from build123d import *

# Parameters (mm, degrees)
F0_W         = 298.45
F0_H         = 457.2
F1_DEPTH     = 19.05
F3_W         = 19.05
F3_H         = 457.2
F4_DEPTH     = 6.35
F5_T1_DEPTH  = 327.025
F5_T3_DEPTH  = 419.1
F5_T5_DEPTH  = 47.625
F5_S9_W      = 19.05
F5_S9_H      = 19.05
F5_T10_DEPTH = 19.05
F5_S15_W     = 19.05
F5_S15_H     = 19.05
F5_T16_DEPTH = 19.05
F6_W         = 19.05
F6_H         = 457.2
F7_DEPTH     = 19.05
F8_W         = 76.2
F8_H         = 19.05
F9_DEPTH     = 6.35


# Not quite as in the source:
# - a fillet or chamfer that OpenCascade refuses, or shapes differently, is made with other operations: its cross-section is extruded or revolved along the edge and cut away or added


with BuildPart() as f1:
    # F0 (on Front) → F1 (new body)
    with BuildSketch(Plane.XZ):
        Rectangle(F0_W, F0_H)
    extrude(amount=-F1_DEPTH)

    # F3 (on face) → F4 (cut)
    with BuildSketch(Plane(origin=(0, 19.05, 0), x_dir=(-1, 0, 0), z_dir=(0, 1, 0))):
        with Locations((-114.3, 0)):
            Rectangle(F3_W, F3_H)
    extrude(amount=-F4_DEPTH, mode=Mode.SUBTRACT)

    # F5: fillet of radius 19.05 on 5 edges, made by hand

    # F5_s2 → F5_t1 (cut)
    with BuildSketch(Plane.YZ.offset(-196.85)):
        with BuildLine():
            ThreePointArc((19.05, -228.6), (5.5796158184, -223.0203841816), (0, -209.55))
            Line((0, -209.55), (0, -228.6))
            Line((0, -228.6), (19.05, -228.6))
        make_face()
        with BuildLine():
            ThreePointArc((19.05, 228.6), (5.5796158184, 223.0203841816), (0, 209.55))
            Line((0, 209.55), (0, 228.6))
            Line((0, 228.6), (19.05, 228.6))
        make_face()
    extrude(amount=F5_T1_DEPTH, mode=Mode.SUBTRACT)

    # F5_s4 → F5_t3 (cut)
    with BuildSketch(Plane.XY.offset(-209.55)):
        with BuildLine():
            ThreePointArc((130.175, 0), (143.6453841816, 5.5796158184), (149.225, 19.05))
            Line((149.225, 19.05), (149.225, 0))
            Line((149.225, 0), (130.175, 0))
        make_face()
    extrude(amount=F5_T3_DEPTH, mode=Mode.SUBTRACT)

    # F5_s6 → F5_t5 (cut)
    with BuildSketch(Plane.XZ.offset(-66.675)):
        with BuildLine():
            ThreePointArc((130.175, -228.6), (143.6453841816, -223.0203841816), (149.225, -209.55))
            Line((149.225, -209.55), (149.225, -228.6))
            Line((149.225, -228.6), (130.175, -228.6))
        make_face()
        with BuildLine():
            ThreePointArc((130.175, 228.6), (143.6453841816, 223.0203841816), (149.225, 209.55))
            Line((149.225, 209.55), (149.225, 228.6))
            Line((149.225, 228.6), (130.175, 228.6))
        make_face()
    extrude(amount=F5_T5_DEPTH, mode=Mode.SUBTRACT)


with BuildPart() as f5_tool8:
    # F5_s9 → F5_t10 (new body)
    with BuildSketch(Plane.YZ.offset(130.175)):
        with Locations((9.525, -219.075)):
            Rectangle(F5_S9_W, F5_S9_H)
    extrude(amount=F5_T10_DEPTH)

    # F5_s11 → F5_t12 (revolve, cut)
    with BuildSketch(Plane(origin=(130.175, 19.05, -209.55), x_dir=(0, 0.7071067812, 0.7071067812), z_dir=(0, 0.7071067812, -0.7071067812))):
        with BuildLine():
            ThreePointArc((0, -19.05), (19.05, 0), (0, 19.05))
            Line((0, 19.05), (0, -19.05))
        make_face()
    revolve(axis=Axis((130.175, 19.05, -209.55), (1, 0, 0)), mode=Mode.SUBTRACT)


with BuildPart() as f1_1:
    add(f1.part)

    # F5_t7: cut F5_tool8
    add(f5_tool8.part, mode=Mode.SUBTRACT)


with BuildPart() as f5_tool14:
    # F5_s15 → F5_t16 (new body)
    with BuildSketch(Plane.YZ.offset(130.175)):
        with Locations((9.525, 219.075)):
            Rectangle(F5_S15_W, F5_S15_H)
    extrude(amount=F5_T16_DEPTH)

    # F5_s17 → F5_t18 (revolve, cut)
    with BuildSketch(Plane(origin=(130.175, 19.05, 209.55), x_dir=(0, 0.7071067812, -0.7071067812), z_dir=(0, -0.7071067812, -0.7071067812))):
        with BuildLine():
            ThreePointArc((0, -19.05), (19.05, 0), (0, 19.05))
            Line((0, 19.05), (0, -19.05))
        make_face()
    revolve(axis=Axis((130.175, 19.05, 209.55), (1, 0, 0)), mode=Mode.SUBTRACT)


with BuildPart() as f1_2:
    add(f1_1.part)

    # F5_t13: cut F5_tool14
    add(f5_tool14.part, mode=Mode.SUBTRACT)

    # F6 (on face) → F7 (join)
    with BuildSketch(Plane(origin=(0, 19.05, 0), x_dir=(-1, 0, 0), z_dir=(0, 1, 0))):
        with Locations((117.475, 0)):
            Rectangle(F6_W, F6_H)
    extrude(amount=F7_DEPTH)

    # F8 (on face) → F9 (cut, through all)
    with BuildSketch(Plane(origin=(0, 19.05, 0), x_dir=(-1, 0, 0), z_dir=(0, 1, 0))):
        with Locations((-66.675, 104.775)):
            Rectangle(F8_W, F8_H)
        with Locations((-66.675, -104.775)):
            Rectangle(F8_W, F8_H)
    extrude(amount=-F9_DEPTH, mode=Mode.SUBTRACT)


solid = f1_2.part
Geometry check sheet. Reference: the model listing, model coordinates, mm. A direction names the side the tool comes from. Give positions to 0.01 mm unless a question says otherwise; leave off trailing zeros. Write each loop counter-clockwise with the first axis right and the second up, starting at its lowest first coordinate (ties: lowest second). Pieces come first, ordered by that corner, then holes. Notation, with made-up numbers: M 8,49.5 L 25,49.5 A12 ccw 25,72.5 Z; hole C 78.25,37.5 d3. An arc over 180 degrees is marked long. One line per question, with ' | ' between items.
1. Cross-section at C-C (y = 29.5). Enter the section's corners in (x, z).
Ans:
outline: M -127,-228.6 L -107.95,-228.6 L -107.95,228.6 L -127,228.6 Z
2. Cross-section at D-D (y = 6). Enter the section's corners in (x, z) (3 decimals), plus the area to 3 significant figures.
Ans:
outline: M -149.225,-223.428 L 130.175,-223.428 A13.878 ccw 144.053,-209.55 L 144.053,209.55 A13.878 ccw 130.175,223.428 L -149.225,223.428 Z | area: 131,000 mm2
3. Cross-section at A-A (z = -80). Enter the section's corners in (x, y) (3 decimals), plus the area to 3 significant figures.
Ans:
outline: M -149.225,0 L 130.175,0 A19.05 ccw 149.225,19.05 L 123.825,19.05 L 123.825,12.7 L 104.775,12.7 L 104.775,19.05 L -107.95,19.05 L -107.95,38.1 L -127,38.1 L -127,19.05 L -149.225,19.05 Z | area: 5,850 mm2
4. Scan lines: line 1 along Y through (x, z) = (49, 178.5); line 2 along X through (y, z) = (35, -189); line 3 along Z through (x, y) = (126.5, 12.5). Record each from-to range of solid material in increasing order. Write a range as from..to.
Ans:
line 1: 0..19.05 | line 2: -127..-107.95 | line 3: -227.44..227.44
5. Cross-section at B-B (x = 62). Enter the section's corners in (y, z), plus the area to 3 significant figures.
Ans:
outline: M 0,-209.55 A19.05 ccw 19.05,-228.6 L 19.05,-114.3 L 12.7,-114.3 L 12.7,-95.25 L 19.05,-95.25 L 19.05,95.25 L 12.7,95.25 L 12.7,114.3 L 19.05,114.3 L 19.05,228.6 A19.05 ccw 0,209.55 Z | area: 8,310 mm2
6. Gauge pin test, flat ends, axial feed: pin 1 (1 mm diameter, centred on x = -34.5, z = 44, fed in from +Y); pin 2 (5 mm diameter, centred on y = 15.5, z = -172.5, fed in from +X); pin 3 (15 mm diameter, centred on y = 24.5, z = -72, fed in from -X) (3 decimals); pin 4 (1.9 mm diameter, centred on x = 77, y = 16, fed in from -Z). Record the tip position at first contact, or that the pin passes through.
Ans:
pin 1: y = 19.05 | pin 2: x = 149.2 | pin 3: x = -149.225 | pin 4: z = -228.48
7. Set-up check for faces 1 (the face through (-138, 19.05, 3)), 2 (the face through (-3, 19.05, 3)), 3 (the face through (-117, 38.1, 3)): record each of +Z, -Z, +X, -X, +Y, -Y from which the full face is reachable in a straight line by a thin tool's end or side.
Ans:
face 1: +Z, -Z, -X, +Y | face 2: +Z, -Z, +X, +Y | face 3: +Z, -Z, +X, -X, +Y
